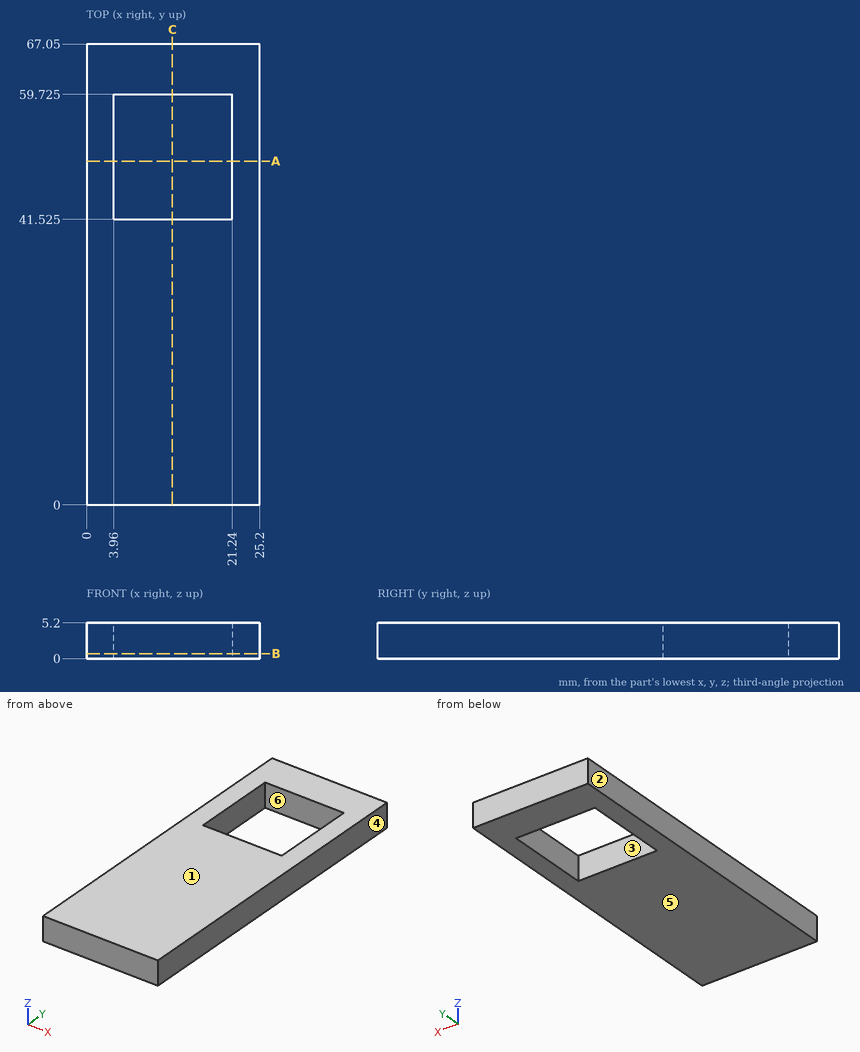
For this review, use the dimensioned drawing (mm, ordinates from the lowest corner) and the shaded views. A direction names the side the tool comes from. Coordinates: 2 decimals unless noted, no trailing zeros. Order: outer loops, then holes, each group sorted by start corner. A loop starts at its lowest first (then second) coordinate and runs counter-clockwise, first axis right, second up. Notation, with made-up numbers: M 43,55.25 L 60,55.25 A15 ccw 60,83.25 Z; hole C 51.25,27.25 d5. An arc over 180 degrees is marked long. Answer as a JSON object with one key per item and string values. Group by question number.
1) Add section A-A, the plane y = 50. Write out the cut boundary in (x, z).
2) Mouldability with a two-part tool opening along X and no side actions: class the marked faces 1, 2, 3 and 4 as pulls with the +X half, pulls with the -X half, needs draft (parallel to the pull), parting line crosses it, or undercut.
3) Add section B-B, the plane z = 0.7. Write out the cut boundary in (x, y) (3 decimals), then the cut area to 3 significant figures.
4) Tool access review of the marked faces 5 and 6: name each direction out of +Z, -Z, +X, -X, +Y, -Y from which nothing blocks a thin tool from reaching the whole face with its end or side.
5) Wall thickness on L1, parallel to Y at x = 12.5, z = 4.7 (3 decimals); L2, parallel to X at y = 47.5, z = 0.2: over which ranges is each line inside the solid? List them lowest first.
6) Add section C-C, the plane x = 12.5. Write out the cut boundary in (y, z) (3 decimals).
Computed values:
{
 "1": {"outline": "M 0,0 L 3.96,0 L 3.96,5.2 L 0,5.2 Z; M 21.24,0 L 25.2,0 L 25.2,5.2 L 21.24,5.2 Z"},
 "2": {"face 1": "needs draft", "face 2": "pulls with the -X half", "face 3": "undercut", "face 4": "pulls with the +X half"},
 "3": {"outline": "M 0,0 L 25.2,0 L 25.2,67.05 L 0,67.05 Z; hole M 3.96,41.525 L 21.24,41.525 L 21.24,59.725 L 3.96,59.725 Z", "area": "1,380 mm^2"},
 "4": {"face 5": "-Z, +X, -X, +Y, -Y", "face 6": "+Z, -Z"},
 "5": {"L1": "y = 0 to 41.525, 59.725 to 67.05", "L2": "x = 0 to 3.96, 21.24 to 25.2"},
 "6": {"outline": "M 0,0 L 41.525,0 L 41.525,5.2 L 0,5.2 Z; M 59.725,0 L 67.05,0 L 67.05,5.2 L 59.725,5.2 Z"}
}
